from build123d import *

# Parameters (mm, degrees)
SKETCH1_R           = 3
BOSS_EXTRUDE3_DEPTH = 5
CHAMFER2_SIZE       = 0.5
CUT_EXTRUDE2_DEPTH  = 2


with BuildPart() as part:
    # Sketch1 → Boss-Extrude3 (new body)
    with BuildSketch(Plane(origin=(0, 0, 0), x_dir=(1, 0, 0), z_dir=(0, 1, 0))):
        Circle(SKETCH1_R)
    extrude(amount=-BOSS_EXTRUDE3_DEPTH)

    # Sketch3 → Revolve2 (revolve)
    with BuildSketch(Plane.XY):
        with BuildLine():
            Line((-5, 0), (-5, 0.3))
            ThreePointArc((-5, 0.3), (-2.969144584, 2.634024216), (0, 3.503635162))
            Line((0, 3.503635162), (0, 0))
            Line((0, 0), (-5, 0))
        make_face()
    revolve(axis=Axis((0, -2, 0), (0, 1, 0)))

    # Chamfer2
    chamfer2_edges = [part.edges().sort_by_distance(p)[0] for p in [
        (-3, -5, 0),
    ]]
    chamfer(chamfer2_edges, length=CHAMFER2_SIZE)

    # Sketch4 → Cut-Extrude2 (cut)
    with BuildSketch(Plane(origin=(0, 3.503635162, 0), x_dir=(1, 0, 0), z_dir=(0, 1, 0))):
        Polygon((0, 2.309401077), (-2, 1.154700538), (-2, -1.154700538), (0, -2.309401077), (2, -1.154700538), (2, 1.154700538), align=None)
    extrude(amount=-CUT_EXTRUDE2_DEPTH, mode=Mode.SUBTRACT)


solid = part.part
Check sheet for the modelled part. Datum: model origin and axes. Units: mm. A direction names the side the tool comes from. Give positions to 0.01 mm unless a question says otherwise; leave off trailing zeros. Loops run counter-clockwise (first coordinate to the right, second up) from the corner with the lowest first, then second, coordinate; pieces in that order, holes last. Notation, with made-up numbers: M -11,67.25 L -7,67.25 A24 ccw -7,106.25 Z; hole C -33,18.25 d3. An arc over 180 degrees is marked long. Use a Markdown table: item, result. Add a question column.
Q1. Sectioned sample at C-C, the plane y = -1.5. Record the cut outline in (x, z), then the cut area to 3 significant figures.
Q2. Sectioned sample at D-D, the plane x = -3.25. Record the cut outline in (y, z).
Q3. Tool access check on faces 5 (the flat face through (0, -5, 0)), 6 (the flat face through (2, 2, 0)). Record the directions out of +Z, -Z, +X, -X, +Y, -Y that give a thin tool (end or side, any length) a straight path to the whole face; none if there is none.
Q4. Sectioned sample at B-B, the plane z = 0. Record the cut outline in (x, y).
Q5. Mould release check, pull along Z, two halves, no side actions. Record for faces 1 (the cylindrical face through (-3, -2, 0)), 2 (the flat face through (-2, 2, 0)), 3 (the flat face through (3.3, 0, 0.1)), 4 (the flat face through (-0.99, 2.33, -1.74)): pulls with the +Z half, pulls with the -Z half, needs draft (parallel to the pull), parting line crosses it, or undercut.
Q6. Go/stop test with flat-tipped pins: pin 1 (4.5 mm diameter, centred on x = 0.5, z = 0, fed in from +Y); pin 2 (4 mm diameter, centred on x = 3.5, y = -2.5, fed in from -Z); pin 3 (1 mm diameter, centred on y = 1, z = -0.5, fed in from -X); pin 4 (0.8 mm diameter, centred on y = 2.5, z = 0, fed in from -X). Record where each tip stops, or that it passes through.
Q7. Sectioned sample at A-A, the plane y = 2.5. Record the cut outline in (x, z), then the cut area to 3 significant figures.
Q8. Scan lines: line 1 along Y through (x, z) = (1.25, 1.5); line 2 along Z through (x, y) = (1.5, 2.75); line 3 along X through (y, z) = (1.75, -2). Record each from-to range of solid material in increasing order. Write a range as [from, to].
Verdict:
| question | item | result |
|---|---|---|
| 1 | outline | C 0,0 d6 |
| 1 | area | 28.3 mm^2 |
| 2 | outline | M 0,-3.8 L 0.3,-3.8 A4.44 ccw 0.3,3.8 L 0,3.8 Z |
| 3 | face 5 | +Z, -Z, +X, -X, -Y |
| 3 | face 6 | +Y |
| 4 | outline | M -5,0 L -3,0 L -3,-4.5 L -2.5,-5 L 2.5,-5 L 3,-4.5 L 3,0 L 5,0 L 5,0.3 A5.5 ccw 2,3.13 L 2,1.5 L -2,1.5 L -2,3.13 A5.5 ccw -5,0.3 Z |
| 5 | face 1 | parting line crosses it |
| 5 | face 2 | undercut |
| 5 | face 3 | needs draft |
| 5 | face 4 | undercut |
| 6 | pin 1 | y = 3.13 |
| 6 | pin 2 | z = -2.6 |
| 6 | pin 3 | x = -4.88 |
| 6 | pin 4 | x = -3.67 |
| 7 | outline | C 0,0 d6.34; hole M -2,-1.15 L 0,-2.31 L 2,-1.15 L 2,1.15 L 0,2.31 L -2,1.15 Z |
| 7 | area | 17.7 mm^2 |
| 8 | line 1 | [-5, 1.5] |
| 8 | line 2 | [-2.34, -1.44], [1.44, 2.34] |
| 8 | line 3 | [-3.5, -0.54], [0.54, 3.5] |
